For this review, use the dimensioned drawing (mm, ordinates from the lowest corner) and the shaded views. A direction names the side the tool comes from. Round coordinates to 2 decimals unless told otherwise and drop trailing zeros. Loops run counter-clockwise (first coordinate to the right, second up) from the corner with the lowest first, then second, coordinate; pieces in that order, holes last. Notation, with made-up numbers: (-33.5, 63) - (-29.5, 63) arc R20 cw to (-29.5, 73) - close; hole circle Ø3 at (38, 13.25). An arc over 180 degrees is marked (long way). Use one line per item in the form item = value. Start each with the question number.
(1) We need section A-A, the plane z = 40. Write out the cut boundary in (x, y), then the cut area to 3 significant figures.
(2) Wall thickness on probe 1 along X at (y, z) = (174, 40); probe 2 along X at (y, z) = (16, 40); probe 3 along Z at (x, y) = (42, 152): over which ranges is each line inside the solid? List them lowest first. Write a range as [from, to].
(3) For pin 1 (24 mm diameter, centred on x = 25.5, z = 35.5, fed in from +Y); pin 2 (8 mm diameter, centred on x = 61.5, y = 261.5, fed in from -Z); pin 3 (3 mm diameter, centred on y = 72, z = 21, fed in from -X); pin 4 (1 mm diameter, centred on x = 15, y = 126.5, fed in from -Z), all flat-tipped, find the tip position at first contact; note any pin that passes through.
(4) Machinability: for the marked faces 1, 2 and 3, which of the approach directions +Z, -Z, +X, -X, +Y, -Y give a long, thin tool a straight path to every point of the face, cutting with its end or side? Answer none if there is none.
(5) We need section D-D, the plane y = 66. Write out the cut boundary in (x, z).
(6) We need section C-C, the plane y = 195. Write out the cut boundary in (x, z).
(7) We need section B-B, the plane x = 40. Write out the cut boundary in (y, z), then the cut area to 3 significant figures.
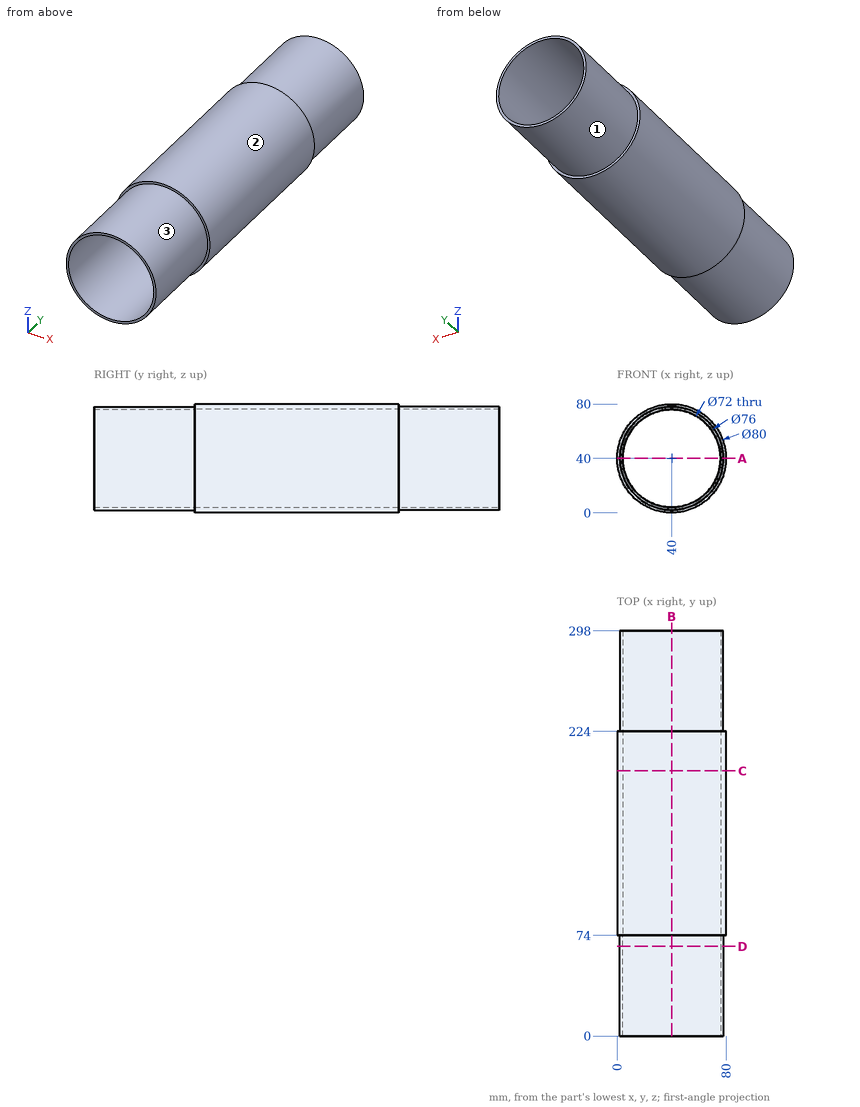
Data:
q1.outline = (0, 74) - (2, 74) - (2, 0) - (4, 0) - (4, 298) - (2, 298) - (2, 224) - (0, 224) - close; (76, 0) - (78, 0) - (78, 74) - (80, 74) - (80, 224) - (78, 224) - (78, 298) - (76, 298) - close
q1.area = 1,790 mm^2
q2.probe_1 = [0, 4], [76, 80]
q2.probe_2 = [2, 4], [76, 78]
q2.probe_3 = [0.05, 4.06], [75.94, 79.95]
q3.pin_1 = through
q3.pin_2 = 6.27
q3.pin_3 = 6.27
q3.pin_4 = 8.38
q4.face_1 = +Y
q4.face_2 = +Y, -Y
q4.face_3 = -Y
q5.outline = circle Ø76 at (40, 40); hole circle Ø72 at (40, 40)
q6.outline = circle Ø80 at (40, 40); hole circle Ø72 at (40, 40)
q7.outline = (0, 2) - (74, 2) - (74, 0) - (224, 0) - (224, 2) - (298, 2) - (298, 4) - (0, 4) - close; (0, 76) - (298, 76) - (298, 78) - (224, 78) - (224, 80) - (74, 80) - (74, 78) - (0, 78) - close
q7.area = 1,790 mm^2
